Part model, mm, in its own coordinate system. A direction names the side the tool comes from. Give positions to 0.01 mm unless a question says otherwise; leave off trailing zeros. Write each loop counter-clockwise with the first axis right and the second up, starting at its lowest first coordinate (ties: lowest second). Pieces come first, ordered by that corner, then holes. Notation, with made-up numbers: M 13.5,-23 L 46.5,-23 A27 ccw 46.5,8 Z; hole C 32,68 d11. An arc over 180 degrees is marked long. Use a Markdown table: item, result.
```python
from build123d import *

# Parameters (mm, degrees)
F0_W        = 192.5
F0_H        = 180
F1_DEPTH    = 1.5
F2_W        = 172.5
F2_H        = 150
F3_DEPTH    = 5.5
F4_T        = 2.5
F4_T3_DEPTH = 155
F4_T5_DEPTH = 177.5
F6_W        = 167.5
F6_H        = 4.5
F7_DEPTH    = 17.501


# Not quite as in the source:
# - a shell that OpenCascade refuses in one call is made with other operations: the cavity is built on its own and cut out


with BuildPart() as f1:
    # F0 (on Front) → F1 (new body)
    with BuildSketch(Plane.XZ):
        Rectangle(F0_W, F0_H)
    extrude(amount=F1_DEPTH)

    # F2 (on face) → F3 (join)
    with BuildSketch(Plane.XZ.offset(1.5)):
        Rectangle(F2_W, F2_H)
    extrude(amount=F3_DEPTH)

    # F4: shell of thickness 2.5, made by hand


with BuildPart() as f4_core1:
    # F4_t2: copy of F1
    add(f1.part)

    # the walls: a layer under each face that stays
    f4_faces = [f4_core1.faces().sort_by_distance(p)[0] for p in [
        (96.25, -0.75, 0),
        (0, -0.75, -90),
        (0, -0.75, 90),
        (-82.5, -1.5, -77.1428571429),
        (-96.25, -0.75, 0),
        (86.25, -4.25, 0),
        (0, -4.25, 75),
        (-86.25, -4.25, 0),
        (0, -4.25, -75),
        (0, -7, 0),
    ]]
    thicken(f4_faces, amount=-F4_T, mode=Mode.SUBTRACT)

    # F4_s4 → F4_t3 (cut)
    with BuildSketch(Plane.XY.offset(-77.5)):
        Polygon((86.275, -1.525), (86.25, 1), (83.75, 1), (83.75, -1.5), align=None)
        Polygon((-86.275, -1.525), (-86.25, 1), (-83.75, 1), (-83.75, -1.5), align=None)
    extrude(amount=F4_T3_DEPTH, mode=Mode.SUBTRACT)

    # F4_s6 → F4_t5 (cut)
    with BuildSketch(Plane.YZ.offset(-88.75)):
        Polygon((-1.525, 75.025), (1, 75), (1, 72.5), (-1.5, 72.5), align=None)
        Polygon((-1.525, -75.025), (1, -75), (1, -72.5), (-1.5, -72.5), align=None)
    extrude(amount=F4_T5_DEPTH, mode=Mode.SUBTRACT)


with BuildPart() as f1_1:
    add(f1.part)

    # what is left inside the walls is the cavity
    f4_cavity = [f4_core1.part.solids().sort_by_distance(p)[0] for p in [
        (0, -0.025, -24.166667),
    ]]
    add(f4_cavity, mode=Mode.SUBTRACT)

    # F6 (on face) → F7 (cut, through all)
    with BuildSketch(Plane(origin=(0, 0, -72.5), x_dir=(1, 0, 0), z_dir=(0, 0, -1))):
        with Locations((0, 2.25)):
            Rectangle(F6_W, F6_H)
    extrude(amount=F7_DEPTH, mode=Mode.SUBTRACT)


solid = f1_1.part
```
1. Cut at C-C, the plane y = -3.25. Give the cut face in (x, z).
Findings below:
| item | result |
|---|---|
| outline | M -86.25,-75 L -83.75,-75 L -83.75,72.5 L 83.75,72.5 L 83.75,-75 L 86.25,-75 L 86.25,75 L -86.25,75 Z |
2. Cut at B-B, the plane x = 65. Give the cut face in (y, z), then the cut area to 3 significant figures.
Findings below:
| item | result |
|---|---|
| outline | M -7,-75 L -4.5,-75 L -4.5,72.5 L 0,72.5 L 0,90 L -1.5,90 L -1.5,75 L -7,75 Z |
| area | 409 mm2 |
3. Tool access for faces 1 (the flat face through (-1, -4, 75)), 2 (the flat face through (-1, -7, 1)), 3 (the flat face through (-1, -4.5, 0)): list every direction of +Z, -Z, +X, -X, +Y, -Y with a clear straight run to the whole face (end or side of a thin tool).
Findings below:
| item | result |
|---|---|
| face 1 | +Z, +X, -X, -Y |
| face 2 | +Z, -Z, +X, -X, -Y |
| face 3 | -Z, +Y |
4. Drop flat-ended pins along their axis: P1, Ø1.3, axis at x = 25, y = -1, coming from the -Z side; P2, Ø1.6, axis at x = -4.5, y = -5, coming from the +Z side; P3, Ø3, axis at y = -5, z = 33, coming from the -X side. Give the stop position or say it passes through.
Findings below:
| item | result |
|---|---|
| P1 | z = 72.5 |
| P2 | z = 75 |
| P3 | x = -86.25 |
5. Drill centre lines: L1, parallel to X at y = -2, z = -39; L2, parallel to X at y = -0.5, z = -44; L3, parallel to Z at x = -69, y = -2.75. Where is each one in solid material? Low to high.
Findings below:
| item | result |
|---|---|
| L1 | -86.25 to -83.75, 83.75 to 86.25 |
| L2 | -96.25 to -83.75, 83.75 to 96.25 |
| L3 | 72.5 to 75 |
6. Two-plate mould, pull along X, no slides. Class faces 4 (the flat face through (86.25, -4, -1)), 5 (the flat face through (83.75, -2, -8)), 6 (the flat face through (0, 0, 74)), 7 (the flat face through (-86.25, -4, -1)): released by +X, released by -X, zero draft, split by the parting line, or undercut.
Findings below:
| item | result |
|---|---|
| face 4 | released by +X |
| face 5 | undercut |
| face 6 | zero draft |
| face 7 | released by -X |
7. Cut at A-A, the plane z = 9.5. Give the cut face in (x, y).
Findings below:
| item | result |
|---|---|
| outline | M -96.25,-1.5 L -86.25,-1.5 L -86.25,-7 L 86.25,-7 L 86.25,-1.5 L 96.25,-1.5 L 96.25,0 L 83.75,0 L 83.75,-4.5 L -83.75,-4.5 L -83.75,0 L -96.25,0 Z |
